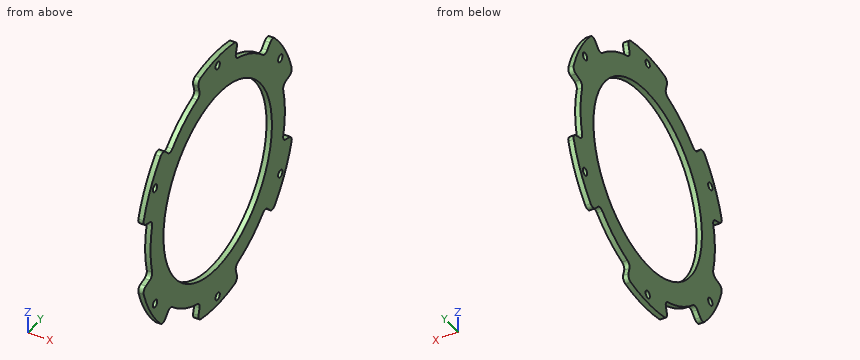
from build123d import *

# Parameters (mm, degrees)
SKETCH_2_R               = 2.807146676
EXTRUDE_2_DEPTH          = 3
SKETCH_3_R               = 52.5
CUT_EXTRUDE_1_DEPTH      = 3
EXTRUDE_START            = -3
SKETCH_4_R               = 2.807146676
SKETCH_4_R_2             = 2.1
EXTRUDE_3_DEPTH          = 3
PATTERN_CIRCULAR_1_COUNT = 6


with BuildPart() as part:
    # 草图2 → 凸台-拉伸2 (new body)
    with BuildSketch(Plane(origin=(0, 0, 0), x_dir=(0, 0, -1), z_dir=(1, 0, 0))):
        with BuildLine():
            Line((-60.415227383, 26.95696902), (-57.584197007, 24.125938644))
            ThreePointArc((-57.584197007, 24.125938644), (-56.706247683, 22.070810886), (-57.492674784, 19.978951059))
            ThreePointArc((-57.492674784, 19.978951059), (-65.839403755, 8.589494146), (-71.529598291, -4.333713637))
            ThreePointArc((-71.529598291, -4.333713637), (-72.947988492, -6.060709399), (-75.166756001, -6.32794686))
            Line((-75.166756001, -6.32794686), (-79.034015413, -5.291717824))
            ThreePointArc((-79.034015413, -5.291717824), (-81.364285194, -5.623240003), (-82.738085883, -7.534453196))
            ThreePointArc((-82.738085883, -7.534453196), (-84.547752509, -23.910505854), (-82.738085883, -40.286558511))
            ThreePointArc((-82.738085883, -40.286558511), (-81.364285194, -42.197771704), (-79.034015413, -42.529293884))
            Line((-79.034015413, -42.529293884), (-75.166756001, -41.493064847))
            ThreePointArc((-75.166756001, -41.493064847), (-72.947988492, -41.760302308), (-71.529598291, -43.48729807))
            ThreePointArc((-71.529598291, -43.48729807), (-65.839403755, -56.410505854), (-57.492674784, -67.799962766))
            ThreePointArc((-57.492674784, -67.799962766), (-56.706247683, -69.891822593), (-57.584197007, -71.946950351))
            Line((-57.584197007, -71.946950351), (-60.415227383, -74.777980727))
            ThreePointArc((-60.415227383, -74.777980727), (-61.293255644, -76.961814644), (-60.324996811, -79.107167538))
            ThreePointArc((-60.324996811, -79.107167538), (-47.047752509, -88.862411137), (-31.960841581, -95.483220195))
            ThreePointArc((-31.960841581, -95.483220195), (-29.618782059, -95.249080495), (-28.16654054, -93.396768757))
            Line((-28.16654054, -93.396768757), (-27.130311503, -89.529509345))
            ThreePointArc((-27.130311503, -89.529509345), (-25.789493318, -87.741619048), (-23.584676016, -87.376754982))
            ThreePointArc((-23.584676016, -87.376754982), (-9.547752509, -88.910505854), (4.489170997, -87.376754982))
            ThreePointArc((4.489170997, -87.376754982), (6.693988299, -87.741619048), (8.034806484, -89.529509345))
            Line((8.034806484, -89.529509345), (9.071035521, -93.396768757))
            ThreePointArc((9.071035521, -93.396768757), (10.52327704, -95.249080495), (12.865336562, -95.483220195))
            ThreePointArc((12.865336562, -95.483220195), (27.952247491, -88.862411137), (41.229491792, -79.107167538))
            ThreePointArc((41.229491792, -79.107167538), (42.197750625, -76.961814644), (41.319722364, -74.777980727))
            Line((41.319722364, -74.777980727), (38.488691988, -71.946950351))
            ThreePointArc((38.488691988, -71.946950351), (37.610742664, -69.891822593), (38.397169765, -67.799962766))
            ThreePointArc((38.397169765, -67.799962766), (46.743898737, -56.410505854), (52.434093272, -43.48729807))
            ThreePointArc((52.434093272, -43.48729807), (53.852483473, -41.760302308), (56.071250982, -41.493064847))
            Line((56.071250982, -41.493064847), (59.938510394, -42.529293884))
            ThreePointArc((59.938510394, -42.529293884), (62.268780175, -42.197771704), (63.642580864, -40.286558511))
            ThreePointArc((63.642580864, -40.286558511), (65.452247491, -23.910505854), (63.642580864, -7.534453196))
            ThreePointArc((63.642580864, -7.534453196), (62.268780175, -5.623240003), (59.938510394, -5.291717824))
            Line((59.938510394, -5.291717824), (56.071250982, -6.32794686))
            ThreePointArc((56.071250982, -6.32794686), (53.852483473, -6.060709399), (52.434093272, -4.333713637))
            ThreePointArc((52.434093272, -4.333713637), (46.743898737, 8.589494146), (38.397169765, 19.978951059))
            ThreePointArc((38.397169765, 19.978951059), (37.610742664, 22.070810886), (38.488691988, 24.125938644))
            Line((38.488691988, 24.125938644), (41.319722364, 26.95696902))
            ThreePointArc((41.319722364, 26.95696902), (42.197750625, 29.140802937), (41.229491792, 31.286155831))
            ThreePointArc((41.229491792, 31.286155831), (27.952247491, 41.04139943), (12.865336562, 47.662208488))
            ThreePointArc((12.865336562, 47.662208488), (10.52327704, 47.428068788), (9.071035521, 45.57575705))
            Line((9.071035521, 45.57575705), (8.034806484, 41.708497638))
            ThreePointArc((8.034806484, 41.708497638), (6.693988299, 39.92060734), (4.489170997, 39.555743275))
            ThreePointArc((4.489170997, 39.555743275), (-9.547752509, 41.089494146), (-23.584676016, 39.555743275))
            ThreePointArc((-23.584676016, 39.555743275), (-25.789493318, 39.92060734), (-27.130311503, 41.708497638))
            Line((-27.130311503, 41.708497638), (-28.16654054, 45.57575705))
            ThreePointArc((-28.16654054, 45.57575705), (-29.618782059, 47.428068788), (-31.960841581, 47.662208488))
            ThreePointArc((-31.960841581, 47.662208488), (-47.047752509, 41.04139943), (-60.324996811, 31.286155831))
            ThreePointArc((-60.324996811, 31.286155831), (-61.293255644, 29.140802937), (-60.415227383, 26.95696902))
        make_face()
        with Locations((-44.547752509, 36.711272411)):
            Circle(SKETCH_2_R, mode=Mode.SUBTRACT)
        with Locations((-79.547752509, -23.910505854)):
            Circle(SKETCH_2_R, mode=Mode.SUBTRACT)
        with Locations((-44.547752509, -84.532284119)):
            Circle(SKETCH_2_R, mode=Mode.SUBTRACT)
        with Locations((25.452247491, -84.532284119)):
            Circle(SKETCH_2_R, mode=Mode.SUBTRACT)
        with Locations((60.452247491, -23.910505854)):
            Circle(SKETCH_2_R, mode=Mode.SUBTRACT)
        with Locations((25.452247491, 36.711272411)):
            Circle(SKETCH_2_R, mode=Mode.SUBTRACT)
    extrude(amount=EXTRUDE_2_DEPTH)

    # 草图3 → 切除-拉伸1 (cut)
    with BuildSketch(Plane(origin=(3, 0, 0), x_dir=(0, 0, -1), z_dir=(1, 0, 0))):
        with Locations((-9.547752509, -23.910505854)):
            Circle(SKETCH_3_R)
    extrude(amount=-CUT_EXTRUDE_1_DEPTH, mode=Mode.SUBTRACT)

    # 草图4 → 凸台-拉伸3 (add)
    with BuildSketch(Plane(origin=(3, 0, 0), x_dir=(0, 0, -1), z_dir=(1, 0, 0)).offset(EXTRUDE_START)):
        with Locations((-44.547752509, 36.711272411)):
            Circle(SKETCH_4_R)
        with Locations((-44.547752509, 36.711272411)):
            Circle(SKETCH_4_R_2, mode=Mode.SUBTRACT)
    extrude_3 = extrude(amount=EXTRUDE_3_DEPTH)

    # 阵列(圆周)1: 凸台-拉伸3 ×6 about axis
    pattern_circular_1_axis = Axis((0, -23.910505854, 9.547752509), (1, 0, 0))
    for i in range(1, PATTERN_CIRCULAR_1_COUNT):
        add(extrude_3.rotate(pattern_circular_1_axis, i * 360 / PATTERN_CIRCULAR_1_COUNT))


solid = part.part
For this review, take the finished solid that the model builds, in its own axes (mm). Round coordinates to 2 decimals unless told otherwise and drop trailing zeros. Order: outer loops, then holes, each group sorted by start corner. A loop starts at its lowest first (then second) coordinate and runs counter-clockwise, first axis right, second up. Notation, with made-up numbers: M 10,-1 L 45,-1 A28 cw 45,36 Z; hole C -21,69.25 d1. An arc over 180 degrees is marked long. Use a Markdown table: item, result. Add a question column.
Item 1: Insertion check: pin 1 (5.5 mm diameter, centred on y = -84.53, z = 44.55, fed in from +X). The pin has a flat end and moves straight along its axis. Give the tip position at first contact, or say it passes through.
Item 2: To check wall thickness, follow line 1 along Y through (x, z) = (2.2, 46); line 2 along Y through (x, z) = (0.45, 13); line 3 along Z through (x, y) = (2.65, -18). State the ranges of each line that lie inside material, in increasing order.
Item 3: Add section C-C, the plane x = 0.65. State how many separate pieces and enclosed holes the cut face has, then the cut area to 3 significant figures.
Item 4: Add section A-A, the plane y = -57.5. Give the boundary of the cut face in (x, z).
Item 5: Add section B-B, the plane z = 40. Give the boundary of the cut face in (x, y).
Item 6: Add section D-D, the plane z = 69. Give the boundary of the cut face in (x, y).
Geometry results:
| question | item | result |
|---|---|---|
| 1 | pin 1 | stops at x = 3 |
| 2 | line 1 | y = -89.46 to -86.05, -83.02 to -61.69, 13.87 to 35.19, 38.23 to 41.64 |
| 2 | line 2 | y = -88.82 to -76.3, 28.48 to 41 |
| 2 | line 3 | z = -65.22 to -42.62, 61.71 to 84.31 |
| 3 | separate pieces | 1 |
| 3 | enclosed holes | 7 |
| 3 | area | 6,730 mm² |
| 4 | outline | M 0,-46.1 L 3,-46.1 L 3,-30.8 L 0,-30.8 Z; M 0,49.9 L 3,49.9 L 3,65.2 L 0,65.2 Z |
| 5 | outline | M 0,-92.45 L 3,-92.45 L 3,-66.68 L 0,-66.68 Z; M 0,18.86 L 3,18.86 L 3,44.63 L 0,44.63 Z |
| 6 | outline | M 0,-50.19 L 3,-50.19 L 3,2.37 L 0,2.37 Z |
